Autodesk Inventor part; units mm, degrees
ref_plane "YZ Plane" through (0, 0, 0) normal (1, 0, 0) x (0, 1, 0)
ref_plane "XZ Plane" through (0, 0, 0) normal (0, 1, 0) x (-1, 0, 0)
ref_plane "XY Plane" through (0, 0, 0) normal (0, 0, 1) x (1, 0, 0)
sketch "Sketch1" plane through (0, 0, 0) normal (0, 0, 1) x (1, 0, 0)
  line L0 (0, 1489.5) -> (-190.7006, 1489.5)
  line L1 (-190.7006, 1489.5) -> (-190.7006, 0)
  line L2 (-190.7006, 0) -> (0, 0)
  line L3 (0, 0) -> (0, 1489.5)
  line L4 (-190.7006, 100) -> (-66, 100)
  line L5 (-66, 100) -> (-66, 105)
  line L6 (-66, 105) -> (-190.7006, 105)
  line L7 (-190.7006, 105) -> (-190.7006, 100)
  line L8 (-190.7006, 596.6667) -> (-66, 596.6667)
  line L9 (-66, 596.6667) -> (-66, 601.6667)
  line L10 (-66, 601.6667) -> (-190.7006, 601.6667)
  line L11 (-190.7006, 601.6667) -> (-190.7006, 596.6667)
  line L12 (-190.7006, 1093.3333) -> (-66, 1093.3333)
  line L13 (-66, 1093.3333) -> (-66, 1098.3333)
  line L14 (-66, 1098.3333) -> (-190.7006, 1098.3333)
  line L15 (-190.7006, 1098.3333) -> (-190.7006, 1093.3333)
  circle A0 centre (-190.7006, 1335) radius 30
  point P0 (-190.7006, 1098.3333)
  point P1 (-190.7006, 1093.3333)
  point P2 (-190.7006, 601.6667)
  point P3 (-190.7006, 596.6667)
  point P4 (-190.7006, 1365)
  point P5 (-190.7006, 1305)
  dimension "d0" = 1489.5
  dimension "d1" = 190.7006
  dimension "d2" = 5
  dimension "d4" = 100
  dimension "d7" = 496.6667
  dimension "d23" = 66
  dimension "d29" = 60
  dimension "d30" = 1335
extrude "Plate1" add sketch "Sketch1" along normal blind 4 contours L3 L2 L1 L4 L5 L6 L8 L9 L10 L12 L13 L14 A0 L0
sketch "Sketch2" plane through (-4, 1489.5, 0) normal (1, 0, 0) x (0, 1, 0)
  line L0 (-1489.5, 0) -> (0, 0)
  line L1 (0, 0) -> (0, 60)
  line L2 (0, 60) -> (-1489.5, 60)
  line L3 (-1489.5, 60) -> (-1489.5, 0)
edge flange "Flange1" height 60 angle 90 thickness 4 bend radius 4 thickness toward (1, 0, 0) relief tear relief width 4 relief depth 2 edges at (0, 744.75, 4) wall of the first edge with corners at (-4, 0, 0) (-4, 1489.5, 0) (-4, 1489.5, 60) (-4, 0, 60)
bend "Bend1"
corner "Corner1"
chamfer "Corner Chamfer1" distance 3 angle 45 6 edges at (-190.7006, 100, 2) (-190.7006, 105, 2) (-190.7006, 596.6667, 2) (-190.7006, 601.6667, 2) (-190.7006, 1098.3333, 2) (-190.7006, 1093.3333, 2)
sketch "Sketch4" plane through (0, 0, 60) normal (1, 0, 0) x (0, 0, -1)
  line L0 (52, 0) -> (52, 1489.5) construction
  line L1 (0, 1489.5) -> (52, 1489.5) construction
  line L2 (0, 0) -> (0, 1489.5) construction
  line L3 (52, 0) -> (0, 0)
  circle A0 centre (18, 1139.5) radius 9
  circle A1 centre (18, 642.8333) radius 9
  circle A2 centre (18, 146.1667) radius 9
  point P0 (60, 0)
  dimension "d31" = 18
  dimension "d32" = 18
  dimension "d33" = 350
  dimension "d36" = 496.6667
extrude "Cut1" cut sketch "Sketch4" against normal blind 4
equation "\"d0\" = Стрингер_длина"
equation "\"d1\" = стрингер_глубина_1"
equation "\"d2\" = паз_под_стрингер_толщина"
equation "\"d7\" = Шаг_шпангоутов"
equation "\"d23\" = паз_под_стрингер_глубина - Thickness"
equation "\"d29\" = 2 * радиус_выреза_под_сварку"
equation "\"d36\" = Шаг_шпангоутов"
equation "\"d41\" = Thickness"
equation "\"d12\" = Thickness"
equation "\"d13\" = BendReliefWidth"
equation "\"d14\" = BendReliefDepth"
equation "\"d15\" = MinimumRemnant"
equation "\"d16\" = TransitionRadius"
equation "\"d17\" = ребро_усилителей"
equation "\"d19\" = BendRadius"
equation "\"d20\" = CornerReliefSize"
equation "\"d21\" = GapSize"
equation "\"d22\" = JacobiRadiusSize"
equation "\"BendRadius\" = Thickness"
equation "\"BendReliefWidth\" = Thickness"
equation "\"BendReliefDepth\" = 0.5 * Thickness"
equation "\"CornerReliefSize\" = 4 * Thickness"
equation "\"MinimumRemnant\" = 2 * Thickness"
equation "\"TransitionRadius\" = BendRadius"
equation "\"JacobiRadiusSize\" = BendRadius"
equation "\"GapSize\" = Thickness"
properties part number "GBK 0102 stringer 1" material "Steel"
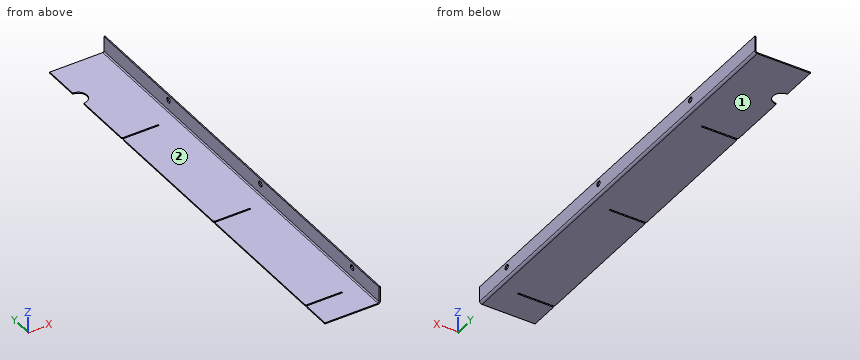
Here's how the part is built. I have some questions about the finished solid (model axes, mm). Face numbers are marked on the shaded views. A direction names the side the tool comes from. Round coordinates to 2 decimals unless told otherwise and drop trailing zeros. Loops run counter-clockwise (first coordinate to the right, second up) from the corner with the lowest first, then second, coordinate; pieces in that order, holes last. Notation, with made-up numbers: (-15, -37.5) -> (6, -37.5) arc R21 ccw to (6, -13.5) -> close; hole circle Ø1 at (34, -36). An arc over 180 degrees is marked (long way). Answer as CSV lines item,"result". Start each with the question number.
1. For the marked faces 1 and 2, which set-ups out of +Z, -Z, +X, -X, +Y, -Y let a thin tool reach every point of the face, with its end or its side?
2. Imagine slicing it at A-A on x = -88.5. Write out the boundary of the cut face in (y, z).
3. Imagine slicing it at B-B on z = 42. Write out the boundary of the cut face in (x, y), plus the area to 3 significant figures.
4. I'm going to push flat-ended pins straight in: P1, Ø3, axis at x = -105, z = 2, coming from the -Y side; P2, Ø12, axis at x = -105.5, y = 572.5, coming from the +Z side; P3, Ø20.5, axis at y = 642.83, z = 42, coming from the -X side; P4, Ø1.2, axis at y = 1096, z = 2, coming from the -X side. Where does each tip first touch, or does it pass through?
5. I need wall thicknesses on probe 1 along Y at (x, z) = (-3, 42); probe 2 along Z at (x, y) = (-170, 1175.5); probe 3 along X at (y, z) = (434, 34). Which ranges of each line are inside material? Lowest first, please. Write a range as from..to.
6. Imagine slicing it at C-C on y = 1335. Write out the boundary of the cut face in (x, z), plus the area to 4 significant figures.
Solution:
1,face 1,"-Z, +X, -X, +Y, -Y"
1,face 2,"+Z, -X, +Y, -Y"
2,outline,"(0, 0) -> (100, 0) -> (100, 4) -> (0, 4) -> close; (105, 0) -> (596.67, 0) -> (596.67, 4) -> (105, 4) -> close; (601.67, 0) -> (1093.33, 0) -> (1093.33, 4) -> (601.67, 4) -> close; (1098.33, 0) -> (1489.5, 0) -> (1489.5, 4) -> (1098.33, 4) -> close"
3,outline,"(-4, 0) -> (0, 0) -> (0, 137.17) -> (-4, 137.17) -> close; (-4, 155.17) -> (0, 155.17) -> (0, 633.83) -> (-4, 633.83) -> close; (-4, 651.83) -> (0, 651.83) -> (0, 1130.5) -> (-4, 1130.5) -> close; (-4, 1148.5) -> (0, 1148.5) -> (0, 1489.5) -> (-4, 1489.5) -> close"
3,area,"5,740 mm²"
4,P1,"y = 0"
4,P2,"z = 4"
4,P3,"x = -4"
4,P4,"x = -66"
5,probe 1,"0..137.17, 155.17..633.83, 651.83..1130.5, 1148.5..1489.5"
5,probe 2,"0..4"
5,probe 3,"-4..0"
6,outline,"(-160.7, 0) -> (-8, 0) arc R8 ccw to (0, 8) -> (0, 60) -> (-4, 60) -> (-4, 8) arc R4 cw to (-8, 4) -> (-160.7, 4) -> close"
6,area,"856.5 mm²"
